Source: CAD feature listing. Evaluate the final solid. Frame: model axes, mm. A direction names the side the tool comes from. Round coordinates to 2 decimals unless told otherwise and drop trailing zeros. Loops run counter-clockwise (first coordinate to the right, second up) from the corner with the lowest first, then second, coordinate; pieces in that order, holes last. Notation, with made-up numbers: M 73,22 L 128,22 A17 cw 128,39 Z; hole C 42.25,85 d7. An arc over 180 degrees is marked long. Answer as a JSON object with one key per item and string values.
from build123d import *

# Parameters (mm, degrees)
PAD_DEPTH     = 5
SKETCH003_R   = 8.028816
SKETCH003_R_2 = 2.5
PAD001_DEPTH  = 1


with BuildPart() as part:
    # Sketch → Pad (new body, symmetric)
    with BuildSketch(Plane.XY):
        with BuildLine():
            ThreePointArc((0, -4.65), (4.573728, -0.838758), (1.65, 4.347413))
            Line((1.65, 6.25), (1.65, 4.347413))
            Line((0, 6.25), (1.65, 6.25))
            Line((0, 13.5), (0, 6.25))
            ThreePointArc((0, -13.5), (13.5, 0), (0, 13.5))
            Line((0, -4.65), (0, -13.5))
        make_face()
    pad = extrude(amount=PAD_DEPTH, both=True)

    # Mirrored: Pad across Sketch V_Axis
    add(pad.mirror(Plane(origin=(0, 0, 0), x_dir=(0, 0, 1), z_dir=(1, 0, 0))))

    # Sketch001 → Groove (revolve, cut)
    with BuildSketch(Plane.YZ):
        Polygon((13.5, 0), (13.5, 2), (12.5, 1.5), (12.5, 0), align=None)
    groove = revolve(axis=Axis((0, 0, 0), (0, 0, 1)), mode=Mode.SUBTRACT)

    # Mirrored001: Groove across Sketch001 H_Axis
    add(groove.mirror(Plane.XY), mode=Mode.SUBTRACT)

    # Sketch003 → Pad001 (join)
    with BuildSketch(Plane.XY.offset(5)):
        Circle(SKETCH003_R)
        Circle(SKETCH003_R_2, mode=Mode.SUBTRACT)
    extrude(amount=-PAD001_DEPTH)


solid = part.part
Item 1: Section A-A on y = 0. Return the cut outline in (x, z), then the cut area to 3 significant figures.
Answer sheet:
{"outline": "M -13.5,-5 L -4.65,-5 L -4.65,4 L -2.5,4 L -2.5,5 L -13.5,5 L -13.5,2 L -12.5,1.5 L -12.5,-1.5 L -13.5,-2 Z; M 2.5,4 L 4.65,4 L 4.65,-5 L 13.5,-5 L 13.5,-2 L 12.5,-1.5 L 12.5,1.5 L 13.5,2 L 13.5,5 L 2.5,5 Z", "area": "174 mm²"}
Item 2: Section B-B on z = 3.5. Return the cut outline in (x, y).
Answer sheet:
{"outline": "C 0,0 d27; hole M -1.65,4.35 A4.65 ccw long 1.65,4.35 L 1.65,6.25 L -1.65,6.25 Z"}
Item 3: Section C-C on z = 0. Return the cut outline in (x, y).
Answer sheet:
{"outline": "C 0,0 d25; hole M -1.65,4.35 A4.65 ccw long 1.65,4.35 L 1.65,6.25 L -1.65,6.25 Z"}
Item 4: Line query: probe 1 along Y at (x, z) = (0, 4.5); probe 2 along Y at (x, z) = (-0.25, 1); probe 3 along Z at (x, y) = (7.5, 10.25). Output: solid intervals per line, ascending. Write a range as from..to.
Answer sheet:
{"probe 1": "y = -13.5..-2.5, 2.5..13.5", "probe 2": "y = -12.5..-4.64, 6.25..12.5", "probe 3": "z = -5..-1.6, 1.6..5"}
Item 5: Pull-direction query (Y, two-part tool) for faces 3 (the flat face through (3, 0, 5)), 4 (the cylindrical face through (-3.755, 11.923, 0.021)), 5 (the cylindrical face through (-0.54, -2.44, 4.51)); classes: pulls with the +Y half, pulls with the -Y half, needs draft (parallel to the pull), parting line crosses it, or undercut.
Answer sheet:
{"face 3": "needs draft", "face 4": "parting line crosses it", "face 5": "undercut"}
Item 6: Access query for faces 1 (the flat face through (0, 6.25, 0)), 2 (the flat face through (0, -6, -5)). Directions: +Z, -Z, +X, -X, +Y, -Y. A direction counts if a zero-diameter tool reaches every point of the face in a straight line with its end or side. Return the directions, or none.
Answer sheet:
{"face 1": "-Z", "face 2": "-Z, +X, -X, +Y, -Y"}
Item 7: Contact query for flat-ended pins moving along their axis: pin 1 Ø0.6 at (y, z) = (5.5, -2.5) entering from +X; pin 2 Ø1.5 at (y, z) = (-4, 2.5) entering from -X; pin 3 Ø2 at (x, z) = (9, 2.5) entering from -Y. Output: stop coordinate, or through.
Answer sheet:
{"pin 1": "stops at x = 12.46", "pin 2": "stops at x = -13.1", "pin 3": "stops at y = -10.87"}
